Job drawing, mm, ordinate dimensions from the low corner. One solid piece. A direction names the side the tool comes from. Round coordinates to 2 decimals unless told otherwise and drop trailing zeros. Write each loop counter-clockwise with the first axis right and the second up, starting at its lowest first coordinate (ties: lowest second). Pieces come first, ordered by that corner, then holes. Notation, with made-up numbers: (-23.5, 56) -> (-1.5, 56) arc R30 ccw to (-1.5, 87) -> close; hole circle Ø7 at (11, -35.5). An arc over 180 degrees is marked (long way). Use CSV: the item, a comma, the result in double quotes. Start each with the question number.
(1) Two-plate mould, pull along Z, no slides. Class the marked faces 1, 2 and 3: released by +Z, released by -Z, zero draft, split by the parting line, or undercut.
(2) Saw through at D-D (x = 20). Give the cut face in (y, z).
(3) Saw through at C-C (z = 6). Give the cut face in (x, y).
(4) Drop flat-ended pins along their axis: pin 1 (12 mm diameter, centred on y = 18, z = 3.5, fed in from -X); pin 2 (4 mm diameter, centred on y = 8.5, z = 21, fed in from +X). Give the stop position or say it passes through.
(5) Probe line 1 (Z direction, x = 47.5, y = 16); line 2 (X direction, y = 1.75, z = 2.5). List the from-to ranges inside material, lowest first. Write a range as [from, to].
(6) Saw through at A-A (y = 7.25). Give the cut face in (x, z).
(7) Which spindle directions (+Z, -Z, +X, -X, +Y, -Y) get a long thin tool onto all of the face, cutting with end or side? Do the marked faces 4 and 5. Say none if no direction does.
(8) Saw through at B-B (x = 141.5). Give the cut face in (y, z).
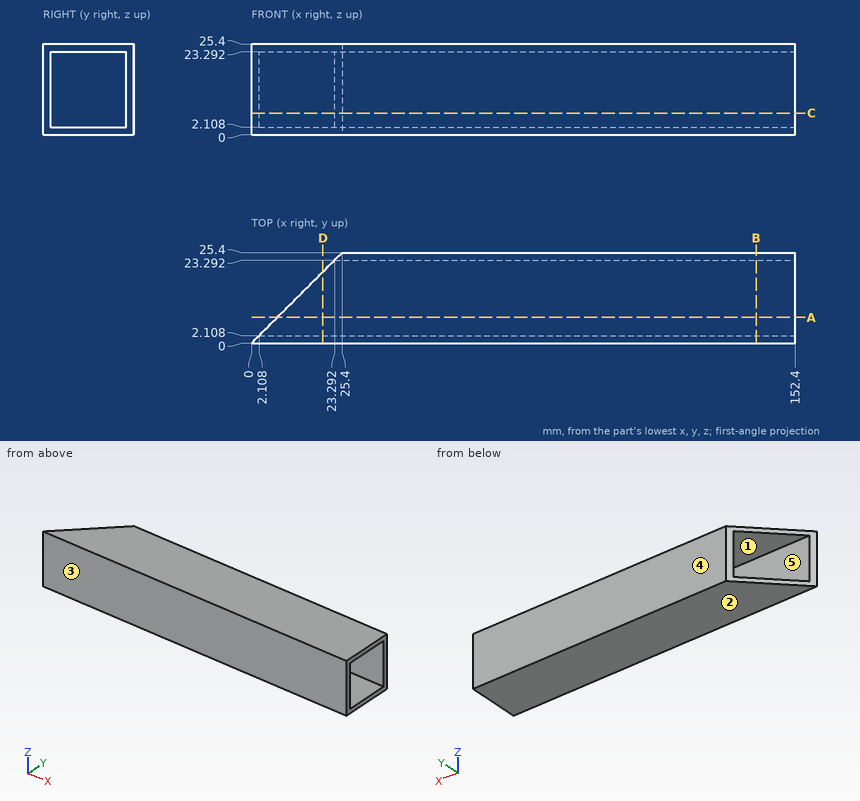
Answers:
1,face 1,"undercut"
1,face 2,"released by -Z"
1,face 3,"zero draft"
2,outline,"(0, 0) -> (20, 0) -> (20, 2.11) -> (2.11, 2.11) -> (2.11, 23.29) -> (20, 23.29) -> (20, 25.4) -> (0, 25.4) -> close"
3,outline,"(0, 0) -> (152.4, 0) -> (152.4, 2.11) -> (2.11, 2.11) -> close; (23.29, 23.29) -> (152.4, 23.29) -> (152.4, 25.4) -> (25.4, 25.4) -> close"
4,pin 1,"stops at x = 12.16"
4,pin 2,"passes through"
5,line 1,"z = [0, 2.11], [23.29, 25.4]"
5,line 2,"x = [1.75, 152.4]"
6,outline,"(7.25, 0) -> (152.4, 0) -> (152.4, 2.11) -> (7.25, 2.11) -> close; (7.25, 23.29) -> (152.4, 23.29) -> (152.4, 25.4) -> (7.25, 25.4) -> close"
7,face 4,"+Z, -Z, +X, -X, +Y"
7,face 5,"+X, -X"
8,outline,"(0, 0) -> (25.4, 0) -> (25.4, 25.4) -> (0, 25.4) -> close; hole (2.11, 2.11) -> (23.29, 2.11) -> (23.29, 23.29) -> (2.11, 23.29) -> close"
